Answer from the drawing. Dimensions are ordinates in mm from the lowest x, y and z of the part. A direction names the side the tool comes from. Give positions to 0.01 mm unless a question says otherwise; leave off trailing zeros. Loops run counter-clockwise (first coordinate to the right, second up) from the corner with the lowest first, then second, coordinate; pieces in that order, holes last. Notation, with made-up numbers: (-5.5, 63.5) - (33.5, 63.5) arc R26 cw to (33.5, 92.5) - close; hole circle Ø8 at (35.25, 52.25). An arc over 180 degrees is marked (long way). Put each result on its own line as item: value. Start each with the question number.
1. A cutting plane is placed at B-B, the plane z = 25. Determine the outline of the cut face in (x, y).
2. A cutting plane is placed at A-A, the plane x = 15. Determine the outline of the cut face in (y, z).
3. A cutting plane is placed at D-D, the plane x = 21. Determine the outline of the cut face in (y, z).
4. For a pull along X with two mould halves and no side action, classify the marked faces 1, 2, 3 and 4 as released by +X, released by -X, zero draft, split by the parting line, or undercut.
5. For the marked faces 5 and 6, determine the directions among +Z, -Z, +X, -X, +Y, -Y from which every point of the face is accessible in a straight line to the end or side of a thin tool.
6. A cutting plane is placed at C-C, the plane y = 4.5. Determine the outline of the cut face in (x, z).
7. Given pin 1 Ø8 at (x, z) = (11, 24) entering from -Y; pin 2 Ø4 at (x, y) = (21, 3) entering from +Z; pin 3 Ø2 at (x, y) = (21.5, 13.5) entering from +Z, each flat-ended and moving along its own axis, determine where each tip first touches the part or whether it passes through.
8. Consider L1, parallel to X at y = 27.75, z = 25; L2, parallel to Y at x = 21.25, z = 21; L3, parallel to Z at x = 17.5, y = 21.5. Determine where each line is inside the solid, lowest interval first. Write a range as from..to.
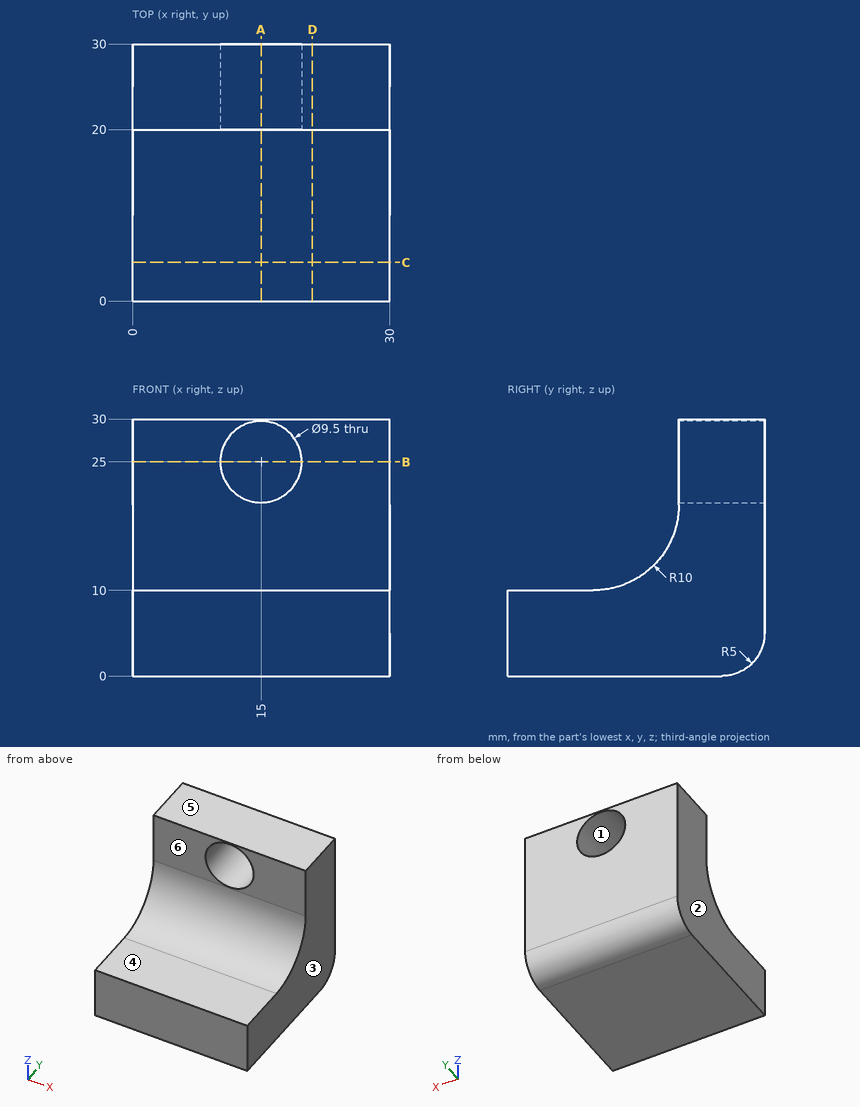
Return value:
1. outline: (0, 20) - (10.25, 20) - (10.25, 30) - (0, 30) - close; (19.75, 20) - (30, 20) - (30, 30) - (19.75, 30) - close
2. outline: (0, 0) - (25, 0) arc R5 ccw to (30, 5) - (30, 20.25) - (20, 20.25) - (20, 20) arc R10 cw to (10, 10) - (0, 10) - close; (20, 29.75) - (30, 29.75) - (30, 30) - (20, 30) - close
3. outline: (0, 0) - (25, 0) arc R5 ccw to (30, 5) - (30, 30) - (20, 30) - (20, 20) arc R10 cw to (10, 10) - (0, 10) - close
4. face 1: undercut
4. face 2: released by -X
4. face 3: released by +X
4. face 4: zero draft
5. face 5: +Z, +X, -X, +Y, -Y
5. face 6: +Z, +X, -X, -Y
6. outline: (0, 0) - (30, 0) - (30, 10) - (0, 10) - close
7. pin 1: stops at y = 20
7. pin 2: stops at z = 10
7. pin 3: stops at z = 11.07
8. L1: x = 0..10.25, 19.75..30
8. L2: y = 20..30
8. L3: z = 0..20.96, 29.04..30
